Source: CAD feature listing. Evaluate the final solid. Frame: model axes, mm. Face numbers are marked on the shaded views. A direction names the side the tool comes from. Round coordinates to 2 decimals unless told otherwise and drop trailing zeros. Order: outer loops, then holes, each group sorted by start corner. A loop starts at its lowest first (then second) coordinate and runs counter-clockwise, first axis right, second up. Notation, with made-up numbers: (10, 87.25) -> (56, 87.25) arc R27 cw to (56, 114.25) -> close; hole circle Ø2 at (12, -2). An arc over 180 degrees is marked (long way). One line per item, written item: value. Start each with the question number.
1) Section B-B (x = 20). Return the cut outline in (y, z).
2) Reachability of the marked faces 1, 2 and 3 from +Z, -Z, +X, -X, +Y, -Y: full face, straight path, thin tool, end or side. Return the list, or none.
3) Section A-A (y = -8.5). Return the cut outline in (x, z).
4) Section D-D (y = -22.5). Return the cut outline in (x, z).
5) Ray query, L1, parallel to Y at x = 48.5, z = 17.5; L2, parallel to Z at x = 37, y = -17.5; L3, parallel to Z at x = 21, y = -16. Return the intervals inside material, ascending.
6) Pin query (flat end, axial travel): P1, Ø6, axis at y = -25, z = 4.5, coming from the -X side. Return the tip coordinate at first contact, or that it passes through.
7) Section C-C (z = 21.5). Return the cut outline in (x, y).
```python
from build123d import *

# Parameters (mm, degrees)
F0_W     = 50.8
F0_H     = 31.75
F1_DEPTH = 31.75
F3_DEPTH = 31.75
F5_DEPTH = 31.75
F7_DEPTH = 12.7


with BuildPart() as f1:
    # F0 (on Front) → F1 (new body)
    with BuildSketch(Plane.XZ):
        with Locations((25.4, 15.875)):
            Rectangle(F0_W, F0_H)
    extrude(amount=F1_DEPTH)

    # F2 (on face) → F3 (cut)
    with BuildSketch(Plane.XZ.offset(31.75)):
        Polygon((50.8, 31.75), (19.05, 31.75), (50.8, 0), align=None)
    extrude(amount=-F3_DEPTH, mode=Mode.SUBTRACT)

    # F4 (on face) → F5 (join)
    with BuildSketch(Plane.XZ.offset(31.75)):
        Polygon((51.5703841816, 18.2796158184), (32.5203841816, 18.2796158184), (50.8, 0), (51.5703841816, 0), align=None)
    extrude(amount=-F5_DEPTH)

    # F6 (on face) → F7 (cut)
    with BuildSketch(Plane.XZ.offset(31.75)):
        Polygon((51.5703841816, 18.2796158184), (32.5203841816, 18.2796158184), (51.5703841816, 0), align=None)
    extrude(amount=-F7_DEPTH, mode=Mode.SUBTRACT)


solid = f1.part
```
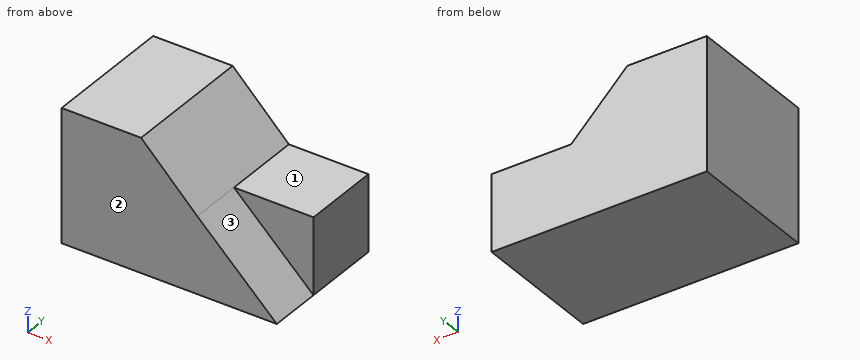
Findings:
1. outline: (-31.75, 0) -> (0, 0) -> (0, 30.8) -> (-31.75, 30.8) -> close
2. face 1: +Z, +X, +Y, -Y
2. face 2: +Z, -Z, +X, -X, -Y
2. face 3: +Z, +X, -Y
3. outline: (0, 0) -> (51.57, 0) -> (51.57, 18.28) -> (32.52, 18.28) -> (19.05, 31.75) -> (0, 31.75) -> close
4. outline: (0, 0) -> (51.57, 0) -> (32.52, 18.28) -> (19.05, 31.75) -> (0, 31.75) -> close
5. L1: -19.05 to 0
5. L2: 0 to 18.28
5. L3: 0 to 29.8
6. P1: x = 0
7. outline: (0, -31.75) -> (29.3, -31.75) -> (29.3, 0) -> (0, 0) -> close
